The listing builds one solid part. Answer for the finished solid, in the listing's coordinates (mm). Face numbers are marked on the shaded views. A direction names the side the tool comes from. Round coordinates to 2 decimals unless told otherwise and drop trailing zeros. Loops run counter-clockwise (first coordinate to the right, second up) from the corner with the lowest first, then second, coordinate; pieces in that order, holes last. Notation, with made-up numbers: (3, 25.25) -> (8, 25.25) arc R15 cw to (8, 44.25) -> close; hole circle Ø4 at (16, 70.25). An arc over 180 degrees is marked (long way). Write each question's results on one line, items separated by ' | '. Start each with the question number.
(1) Straight lines are drawn through the part: probe 1 along Z at (x, y) = (0, -4.85); probe 2 along Z at (x, y) = (9, -3); probe 3 along X at (y, z) = (-5.7, 12.45). For each, find the intervals that lie inside material, in ascending order.
(2) The part is cut by section B-B (x = 0). Determine the outline of the cut face in (y, z), plus the area to 3 significant figures.
(3) The part is cut by section C-C (z = 6.5). Determine the outline of the cut face in (x, y), plus the area to 3 significant figures.
(4) The part is cut by section D-D (y = -5.5). Determine the outline of the cut face in (x, z).
(5) Determine the mould class of the marked faces 1, 2 and 3 for opening direction Z: released by +Z, released by -Z, zero draft, split by the parting line, or undercut.
(6) For the marked faces 4, 5, 6, 7 and 8, determine the directions among +Z, -Z, +X, -X, +Y, -Y from which every point of the face is accessible in a straight line to the end or side of a thin tool.
(7) Flat-ended cylindrical pins translate along their axes: pin 1 (1 mm diameter, centred on y = -1, z = -15.5, fed in from -X); pin 2 (1.9 mm diameter, centred on y = -2, z = -18, fed in from +X); pin 3 (3 mm diameter, centred on x = 9.5, y = -3, fed in from -Z). Find the tip coordinate at first contact, or state that the pin passes through.
(8) The part is cut by section A-A (x = 8). Determine the outline of the cut face in (y, z), plus the area to 3 significant figures.
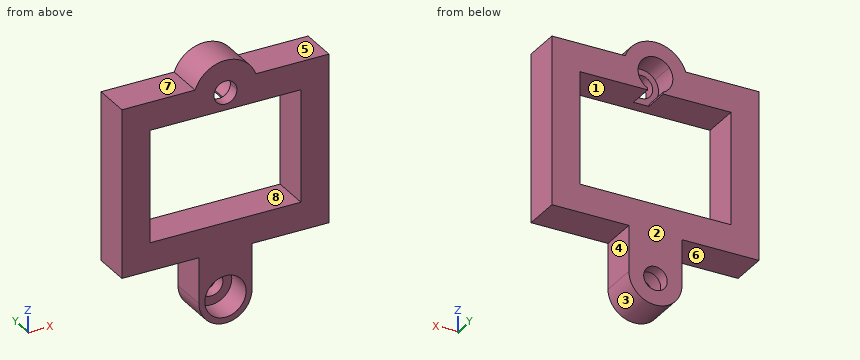
```python
from build123d import *

# Parameters (mm, degrees)
F0_R     = 3.5
F1_DEPTH = 6.35
F0_R_2   = 2
F2_DEPTH = 2
F4_DEPTH = 4.35


with BuildPart() as f1:
    # F0 (on Front) → F1 (new body)
    with BuildSketch(Plane.XZ):
        with BuildLine():
            ThreePointArc((2.95, 12.45), (2.0859650045, 10.3640349955), (0, 9.5))
            ThreePointArc((0, 9.5), (-2.6469321865, 11.1475983722), (-2.3371991785, 14.25))
            Line((-2.3371991785, 14.25), (-5.144171459, 14.25))
            Line((-5.144171459, 14.25), (-17.55, 14.25))
            Line((-17.55, 14.25), (-17.55, -14.25))
            Line((-17.55, -14.25), (-4.5, -14.25))
            Line((-4.5, -14.25), (4.5, -14.25))
            Line((4.5, -14.25), (17.55, -14.25))
            Line((17.55, -14.25), (17.55, 14.25))
            Line((17.55, 14.25), (5.144171459, 14.25))
            Line((5.144171459, 14.25), (2.3371991785, 14.25))
            ThreePointArc((2.3371991785, 14.25), (2.7926007212, 13.4007266756), (2.95, 12.45))
        make_face()
        Polygon((-12.8, -9.5), (-12.8, 9.5), (0, 9.5), (12.8, 9.5), (12.8, -9.5), align=None, mode=Mode.SUBTRACT)
        with BuildLine():
            ThreePointArc((-2.3371991785, 14.25), (-2.6469321865, 11.1475983722), (0, 9.5))
            ThreePointArc((0, 9.5), (2.0859650045, 10.3640349955), (2.95, 12.45))
            ThreePointArc((2.95, 12.45), (2.7926007212, 13.4007266756), (2.3371991785, 14.25))
            Line((2.3371991785, 14.25), (0.75, 14.25))
            ThreePointArc((0.75, 14.25), (1.622498074, 13.5316653826), (1.95, 12.45))
            ThreePointArc((1.95, 12.45), (-1.0816653826, 10.827501926), (-0.75, 14.25))
            Line((-0.75, 14.25), (-2.3371991785, 14.25))
        make_face()
        with BuildLine():
            Line((-5.144171459, 14.25), (-2.3371991785, 14.25))
            ThreePointArc((-2.3371991785, 14.25), (0, 15.4), (2.3371991785, 14.25))
            Line((2.3371991785, 14.25), (5.144171459, 14.25))
            ThreePointArc((5.144171459, 14.25), (0, 17.9), (-5.144171459, 14.25))
        make_face()
        with BuildLine():
            ThreePointArc((2.3371991785, 14.25), (0, 15.4), (-2.3371991785, 14.25))
            Line((-2.3371991785, 14.25), (-0.75, 14.25))
            ThreePointArc((-0.75, 14.25), (0, 14.4), (0.75, 14.25))
            Line((0.75, 14.25), (2.3371991785, 14.25))
        make_face()
        with BuildLine():
            Line((4.5, -14.25), (-4.5, -14.25))
            Line((-4.5, -14.25), (-4.5, -22))
            ThreePointArc((-4.5, -22), (0, -26.5), (4.5, -22))
            Line((4.5, -22), (4.5, -14.25))
        make_face()
        with Locations((0, -22)):
            Circle(F0_R, mode=Mode.SUBTRACT)
    extrude(amount=F1_DEPTH)

    # F0 (on Front) → F2 (join)
    with BuildSketch(Plane.XZ):
        with Locations((0, -22)):
            Circle(F0_R)
        with Locations((0, -22)):
            Circle(F0_R_2, mode=Mode.SUBTRACT)
    extrude(amount=F2_DEPTH)

    # F0 (on Front) + F3 (on face) → F4 (cut)
    with BuildSketch(Plane.XZ):
        with BuildLine():
            ThreePointArc((-2.3371991785, 14.25), (-2.6469321865, 11.1475983722), (0, 9.5))
            ThreePointArc((0, 9.5), (2.0859650045, 10.3640349955), (2.95, 12.45))
            ThreePointArc((2.95, 12.45), (2.7926007212, 13.4007266756), (2.3371991785, 14.25))
            Line((2.3371991785, 14.25), (0.75, 14.25))
            ThreePointArc((0.75, 14.25), (1.622498074, 13.5316653826), (1.95, 12.45))
            ThreePointArc((1.95, 12.45), (-1.0816653826, 10.827501926), (-0.75, 14.25))
            Line((-0.75, 14.25), (-2.3371991785, 14.25))
        make_face()
        with BuildLine():
            ThreePointArc((2.3371991785, 14.25), (0, 15.4), (-2.3371991785, 14.25))
            Line((-2.3371991785, 14.25), (-0.75, 14.25))
            ThreePointArc((-0.75, 14.25), (0, 14.4), (0.75, 14.25))
            Line((0.75, 14.25), (2.3371991785, 14.25))
        make_face()
    with BuildSketch(Plane.XZ):
        with BuildLine():
            Line((-1.3135344248, 9.5), (0, 9.5))
            ThreePointArc((0, 9.5), (-0.6746464011, 9.5781796307), (-1.3135344248, 9.8085747569))
            Line((-1.3135344248, 9.8085747569), (-1.3135344248, 9.5))
        make_face()
        with BuildLine():
            Line((1.3135344248, 9.5), (1.3135344248, 9.8085747569))
            ThreePointArc((1.3135344248, 9.8085747569), (0.6746464011, 9.5781796307), (0, 9.5))
            Line((0, 9.5), (1.3135344248, 9.5))
        make_face()
    extrude(amount=F4_DEPTH, mode=Mode.SUBTRACT)


solid = f1.part
```
Checked values:
1) probe 1: z = -26.5 to -25.5, -18.5 to -9.5, 9.5 to 10.5, 14.4 to 17.9 | probe 2: z = -14.25 to -9.5, 9.5 to 14.25 | probe 3: x = -17.55 to -1.95, 1.95 to 17.55
2) outline: (-6.35, -26.5) -> (0, -26.5) -> (0, -24) -> (-2, -24) -> (-2, -25.5) -> (-6.35, -25.5) -> close; (-6.35, -18.5) -> (-2, -18.5) -> (-2, -20) -> (0, -20) -> (0, -9.5) -> (-6.35, -9.5) -> close; (-6.35, 9.5) -> (-4.35, 9.5) -> (-4.35, 10.5) -> (-6.35, 10.5) -> close; (-6.35, 14.4) -> (-4.35, 14.4) -> (-4.35, 15.4) -> (0, 15.4) -> (0, 17.9) -> (-6.35, 17.9) -> close | area: 89.4 mm2
3) outline: (-17.55, -6.35) -> (-12.8, -6.35) -> (-12.8, 0) -> (-17.55, 0) -> close; (12.8, -6.35) -> (17.55, -6.35) -> (17.55, 0) -> (12.8, 0) -> close | area: 60.3 mm2
4) outline: (-17.55, -14.25) -> (-4.5, -14.25) -> (-4.5, -22) arc R4.5 ccw to (4.5, -22) -> (4.5, -14.25) -> (17.55, -14.25) -> (17.55, 14.25) -> (5.14, 14.25) arc R5.45 ccw to (-5.14, 14.25) -> (-17.55, 14.25) -> close; hole (-12.8, -9.5) -> (12.8, -9.5) -> (12.8, 9.5) -> (-12.8, 9.5) -> close; hole circle Ø7 at (0, -22); hole circle Ø3.9 at (0, 12.45)
5) face 1: undercut | face 2: zero draft | face 3: released by -Z
6) face 4: -Z, +X, +Y, -Y | face 5: +Z, +X, +Y, -Y | face 6: -Z, -X, +Y, -Y | face 7: +Z, -X, +Y, -Y | face 8: +Y, -Y
7) pin 1: stops at x = -4.5 | pin 2: stops at x = 4.5 | pin 3: stops at z = -14.25
8) outline: (-6.35, -14.25) -> (0, -14.25) -> (0, -9.5) -> (-6.35, -9.5) -> close; (-6.35, 9.5) -> (0, 9.5) -> (0, 14.25) -> (-6.35, 14.25) -> close | area: 60.3 mm2
